Read the model definition and answer for the solid it produces. Units are mm, in the model's axes. Coordinates: 2 decimals unless noted, no trailing zeros. Loops run counter-clockwise (first coordinate to the right, second up) from the corner with the lowest first, then second, coordinate; pieces in that order, holes last.
Q1. Straight lines are drawn through the part: line 1 (X direction, y = 2, z = 4.5); line 2 (X direction, y = 2.8, z = 1); line 3 (Z direction, x = -87, y = 0.95). For each, find the intervals that lie inside material, in ascending order.
Q2. Flat-ended cylindrical pins translate along their axes: P1, Ø4, axis at x = -41, z = -5, coming from the -Y side; P2, Ø1.5, axis at x = 61, y = 1, coming from the +Z side; P3, Ø1, axis at y = 2, z = -11, coming from the -X side; P4, Ø0.9, axis at x = -100.5, y = 1, coming from the -Z side. Find the tip coordinate at first contact, or state that the pin passes through.
Q3. Section A-A (y = 1.3) is taken. Count the separate pieces of the cut face and the enclosed holes in it, then the cut area to 3 significant figures.
Q4. Section B-B (x = 69) is taken. Give the vertices of the cut face in (y, z).
from build123d import *

# Parameters (mm, degrees)
SKETCH_1_R          = 1.6
EXTRUDE_1_DEPTH     = 3
SKETCH_3_R          = 1.6
CUT_EXTRUDE_1_DEPTH = 92.290744328
FILLET_1_R          = 1
SKETCH_4_W          = 12
SKETCH_4_H          = 3
CUT_EXTRUDE_2_DEPTH = 92.290744328
SKETCH_5_R          = 1
CUT_EXTRUDE_3_DEPTH = 92.290744328
CUT_EXTRUDE_4_DEPTH = 92.290744328
SKETCH_7_W          = 37
SKETCH_7_H          = 16
SKETCH_7_W_2        = 3
SKETCH_7_H_2        = 9
EXTRUDE_2_DEPTH     = 3
SKETCH_8_R          = 1
CUT_EXTRUDE_5_DEPTH = 128.917942447
FILLET_3_R          = 2


with BuildPart() as part:
    # 草图1 → 凸台-拉伸1 (new body)
    with BuildSketch(Plane(origin=(0, 0, 0), x_dir=(1, 0, 0), z_dir=(0, 1, 0))):
        Polygon((-90, -15), (-72.5, -15), (-72.5, 0.5), (72.5, 0.5), (72.5, -15), (90, -15), (90, 15), (-90, 15), align=None)
        with Locations(Location((78, -10, 0), (0, 0, 270))):
            Circle(SKETCH_1_R, mode=Mode.SUBTRACT)
        with Locations(Location((-78, -10, 0), (0, 0, 90))):
            Circle(SKETCH_1_R, mode=Mode.SUBTRACT)
        with Locations(Location((-83, 10, 0), (0, 0, 270))):
            Circle(SKETCH_1_R, mode=Mode.SUBTRACT)
        with Locations(Location((83, 10, 0), (0, 0, 90))):
            Circle(SKETCH_1_R, mode=Mode.SUBTRACT)
    extrude(amount=EXTRUDE_1_DEPTH)

    # 草图3 → 切除-拉伸1 (cut, through all)
    with BuildSketch(Plane(origin=(0, 3, 0), x_dir=(1, 0, 0), z_dir=(0, 1, 0))):
        with Locations(Location((87, -4.5, 0), (0, 0, 90))):
            Circle(SKETCH_3_R)
        with Locations(Location((-87, -4.5, 0), (0, 0, 270))):
            Circle(SKETCH_3_R)
    extrude(amount=-CUT_EXTRUDE_1_DEPTH, mode=Mode.SUBTRACT)

    # 圆角1
    fillet_1_edges = [part.edges().sort_by_distance(p)[0] for p in [
        (72.5, 1.5, -0.5),
        (-72.5, 1.5, -0.5),
    ]]
    fillet(fillet_1_edges, radius=FILLET_1_R)

    # 草图4 → 切除-拉伸2 (cut, through all)
    with BuildSketch(Plane.XZ):
        with Locations((60, -7.5)):
            Rectangle(SKETCH_4_W, SKETCH_4_H)
        with Locations((30, -7.5)):
            Rectangle(SKETCH_4_W, SKETCH_4_H)
        with Locations((0, -7.5)):
            Rectangle(SKETCH_4_W, SKETCH_4_H)
        with Locations((-30, -7.5)):
            Rectangle(SKETCH_4_W, SKETCH_4_H)
        with Locations((-60, -7.5)):
            Rectangle(SKETCH_4_W, SKETCH_4_H)
    extrude(amount=-CUT_EXTRUDE_2_DEPTH, mode=Mode.SUBTRACT)

    # 草图5 → 切除-拉伸3 (cut, through all)
    with BuildSketch(Plane.XZ):
        with Locations((65, -9)):
            Circle(SKETCH_5_R)
        with Locations((55, -9)):
            Circle(SKETCH_5_R)
        with Locations((55, -6)):
            Circle(SKETCH_5_R)
        with Locations((65, -6)):
            Circle(SKETCH_5_R)
        with Locations((35, -9)):
            Circle(SKETCH_5_R)
        with Locations((25, -9)):
            Circle(SKETCH_5_R)
        with Locations((25, -6)):
            Circle(SKETCH_5_R)
        with Locations((35, -6)):
            Circle(SKETCH_5_R)
        with Locations((5, -9)):
            Circle(SKETCH_5_R)
        with Locations((-5, -9)):
            Circle(SKETCH_5_R)
        with Locations((-5, -6)):
            Circle(SKETCH_5_R)
        with Locations((5, -6)):
            Circle(SKETCH_5_R)
        with Locations((-25, -9)):
            Circle(SKETCH_5_R)
        with Locations((-35, -9)):
            Circle(SKETCH_5_R)
        with Locations((-35, -6)):
            Circle(SKETCH_5_R)
        with Locations((-25, -6)):
            Circle(SKETCH_5_R)
        with Locations((-55, -9)):
            Circle(SKETCH_5_R)
        with Locations((-65, -9)):
            Circle(SKETCH_5_R)
        with Locations((-65, -6)):
            Circle(SKETCH_5_R)
        with Locations((-55, -6)):
            Circle(SKETCH_5_R)
    extrude(amount=-CUT_EXTRUDE_3_DEPTH, mode=Mode.SUBTRACT)

    # 草图6 → 切除-拉伸4 (cut, through all)
    with BuildSketch(Plane.XZ):
        with BuildLine():
            Line((36.1, -9), (36.1, -6))
            ThreePointArc((36.1, -6), (35.050051841, -4.901139311), (33.904554885, -5.9))
            Line((33.904554885, -5.9), (26.095445115, -5.9))
            ThreePointArc((26.095445115, -5.9), (24.949948159, -4.901139311), (23.9, -6))
            Line((23.9, -6), (23.9, -9))
            ThreePointArc((23.9, -9), (24.949948159, -10.098860689), (26.095445115, -9.1))
            Line((26.095445115, -9.1), (33.904554885, -9.1))
            ThreePointArc((33.904554885, -9.1), (35.050051841, -10.098860689), (36.1, -9))
        make_face()
        with BuildLine():
            Line((66.1, -9), (66.1, -6))
            ThreePointArc((66.1, -6), (65.050051841, -4.901139311), (63.904554885, -5.9))
            Line((63.904554885, -5.9), (56.095445115, -5.9))
            ThreePointArc((56.095445115, -5.9), (54.949948159, -4.901139311), (53.9, -6))
            Line((53.9, -6), (53.9, -9))
            ThreePointArc((53.9, -9), (54.949948159, -10.098860689), (56.095445115, -9.1))
            Line((56.095445115, -9.1), (63.904554885, -9.1))
            ThreePointArc((63.904554885, -9.1), (65.050051841, -10.098860689), (66.1, -9))
        make_face()
        with BuildLine():
            Line((6.1, -9), (6.1, -6))
            ThreePointArc((6.1, -6), (5.050051841, -4.901139311), (3.904554885, -5.9))
            Line((3.904554885, -5.9), (-3.904554885, -5.9))
            ThreePointArc((-3.904554885, -5.9), (-5.050051841, -4.901139311), (-6.1, -6))
            Line((-6.1, -6), (-6.1, -9))
            ThreePointArc((-6.1, -9), (-5.050051841, -10.098860689), (-3.904554885, -9.1))
            Line((-3.904554885, -9.1), (3.904554885, -9.1))
            ThreePointArc((3.904554885, -9.1), (5.050051841, -10.098860689), (6.1, -9))
        make_face()
        with BuildLine():
            Line((-23.9, -9), (-23.9, -6))
            ThreePointArc((-23.9, -6), (-24.949948159, -4.901139311), (-26.095445115, -5.9))
            Line((-26.095445115, -5.9), (-33.904554885, -5.9))
            ThreePointArc((-33.904554885, -5.9), (-35.050051841, -4.901139311), (-36.1, -6))
            Line((-36.1, -6), (-36.1, -9))
            ThreePointArc((-36.1, -9), (-35.050051841, -10.098860689), (-33.904554885, -9.1))
            Line((-33.904554885, -9.1), (-26.095445115, -9.1))
            ThreePointArc((-26.095445115, -9.1), (-24.949948159, -10.098860689), (-23.9, -9))
        make_face()
        with BuildLine():
            Line((-53.9, -9), (-53.9, -6))
            ThreePointArc((-53.9, -6), (-54.949948159, -4.901139311), (-56.095445115, -5.9))
            Line((-56.095445115, -5.9), (-63.904554885, -5.9))
            ThreePointArc((-63.904554885, -5.9), (-65.050051841, -4.901139311), (-66.1, -6))
            Line((-66.1, -6), (-66.1, -9))
            ThreePointArc((-66.1, -9), (-65.050051841, -10.098860689), (-63.904554885, -9.1))
            Line((-63.904554885, -9.1), (-56.095445115, -9.1))
            ThreePointArc((-56.095445115, -9.1), (-54.949948159, -10.098860689), (-53.9, -9))
        make_face()
    extrude(amount=-CUT_EXTRUDE_4_DEPTH, mode=Mode.SUBTRACT)

    # 草图7 → 凸台-拉伸2 (add)
    with BuildSketch(Plane.XZ):
        with Locations((-108.5, 2.75)):
            Rectangle(SKETCH_7_W, SKETCH_7_H)
        with Locations((-122.5, 2.75)):
            Rectangle(SKETCH_7_W_2, SKETCH_7_H_2, mode=Mode.SUBTRACT)
    extrude(amount=-EXTRUDE_2_DEPTH)

    # 草图8 → 切除-拉伸5 (cut, through all)
    with BuildSketch(Plane(origin=(0, 3, 0), x_dir=(1, 0, 0), z_dir=(0, 1, 0))):
        with Locations((-123.5025, 0.882536024)):
            Circle(SKETCH_8_R)
        with Locations((-121.4975, 0.882536024)):
            Circle(SKETCH_8_R)
        with Locations((-121.4975, -6.382536024)):
            Circle(SKETCH_8_R)
        with Locations((-123.5025, -6.382536024)):
            Circle(SKETCH_8_R)
    extrude(amount=-CUT_EXTRUDE_5_DEPTH, mode=Mode.SUBTRACT)

    # 圆角3
    fillet_3_edges = [part.edges().sort_by_distance(p)[0] for p in [
        (90, 1.5, 15),
        (72.5, 1.5, 15),
        (-72.5, 1.5, 15),
        (-90, 1.5, 15),
        (-90, 1.5, -15),
        (90, 1.5, -15),
        (-127, 1.5, 10.75),
        (-127, 1.5, -5.25),
        (-90, 1.5, -5.25),
        (-90, 1.5, 10.75),
    ]]
    fillet(fillet_3_edges, radius=FILLET_3_R)


solid = part.part
Numbers:
1. line 1: x = -127 to -124, -121 to -88.6, -85.4 to -72.5, 72.5 to 85.4, 88.6 to 90
1. line 2: x = -127 to -124, -121 to -72.5, 72.5 to 90
1. line 3: z = -15 to 2.9, 6.1 to 15
2. P1: stops at y = 0
2. P2: stops at z = -0.5
2. P3: stops at x = -90
2. P4: stops at z = -5.25
3. separate pieces: 1
3. enclosed holes: 12
3. area: 3,430 mm2
4. outline: (0, -15) - (3, -15) - (3, -0.5) - (0, -0.5) - close
